Work out the finished part from the listing and answer in its coordinate system (mm). A direction names the side the tool comes from. Give positions to 0.01 mm unless a question says otherwise; leave off trailing zeros. Order: outer loops, then holes, each group sorted by start corner. A loop starts at its lowest first (then second) coordinate and runs counter-clockwise, first axis right, second up.
```python
from build123d import *

# Parameters (mm, degrees)
SKETCH_1_W          = 82
SKETCH_1_H          = 82
SKETCH_1_R          = 35.5
EXTRUDE_1_DEPTH     = 315
SKETCH_2_W          = 82
SKETCH_2_H          = 82
EXTRUDE_2_DEPTH     = 35
SKETCH_3_W          = 8
SKETCH_3_H          = 20
CUT_EXTRUDE_1_DEPTH = 315
SKETCH_4_R          = 4
CUT_EXTRUDE_2_DEPTH = 20
FILLET_2_R          = 3
FILLET_3_R          = 3
FILLET_4_R          = 3
FILLET_5_R          = 3
CUT_EXTRUDE_3_DEPTH = 12
SKETCH_6_W          = 29.4
SKETCH_6_H          = 3
CUT_EXTRUDE_4_DEPTH = 10


with BuildPart() as part:
    # 草圖1 → 填料-伸長1 (new body)
    with BuildSketch(Plane.XY):
        Rectangle(SKETCH_1_W, SKETCH_1_H)
        Circle(SKETCH_1_R, mode=Mode.SUBTRACT)
    extrude(amount=EXTRUDE_1_DEPTH)

    # 草圖2 → 填料-伸長2 (add)
    with BuildSketch(Plane(origin=(0, 0, 0), x_dir=(-1, 0, 0), z_dir=(0, 0, -1))):
        Rectangle(SKETCH_2_W, SKETCH_2_H)
    extrude(amount=EXTRUDE_2_DEPTH)

    # 草圖3 → 除料-伸長1 (cut)
    with BuildSketch(Plane.XY.offset(315)):
        with Locations((-37, 0)):
            Rectangle(SKETCH_3_W, SKETCH_3_H)
    extrude(amount=-CUT_EXTRUDE_1_DEPTH, mode=Mode.SUBTRACT)

    # 草圖4 → 除料-伸長2 (cut)
    with BuildSketch(Plane.XY.offset(315)):
        with Locations((-32.9, 33)):
            Circle(SKETCH_4_R)
        with Locations((33.1, 32.9)):
            Circle(SKETCH_4_R)
        with Locations((33, -33.1)):
            Circle(SKETCH_4_R)
        with Locations((-33, -33)):
            Circle(SKETCH_4_R)
    extrude(amount=-CUT_EXTRUDE_2_DEPTH, mode=Mode.SUBTRACT)

    # 圓角2
    fillet_2_edges = [part.edges().sort_by_distance(p)[0] for p in [
        (-36.9, 33, 295),
    ]]
    fillet(fillet_2_edges, radius=FILLET_2_R)

    # 圓角3
    fillet_3_edges = [part.edges().sort_by_distance(p)[0] for p in [
        (29.1, 32.9, 295),
    ]]
    fillet(fillet_3_edges, radius=FILLET_3_R)

    # 圓角4
    fillet_4_edges = [part.edges().sort_by_distance(p)[0] for p in [
        (-37, -33, 295),
    ]]
    fillet(fillet_4_edges, radius=FILLET_4_R)

    # 圓角5
    fillet_5_edges = [part.edges().sort_by_distance(p)[0] for p in [
        (29, -33.1, 295),
    ]]
    fillet(fillet_5_edges, radius=FILLET_5_R)

    # 草圖5 → 除料-伸長3 (cut)
    with BuildSketch(Plane(origin=(0, 41, 0), x_dir=(1, 0, 0), z_dir=(0, 1, 0))):
        with BuildLine():
            Line((-39, 5), (-39, 30))
            ThreePointArc((-39, 30), (-36.8, 32.2), (-34.6, 30))
            Line((-34.6, 30), (-34.6, 5))
            ThreePointArc((-34.6, 5), (-36.8, 2.8), (-39, 5))
        make_face()
    extrude(amount=-CUT_EXTRUDE_3_DEPTH, mode=Mode.SUBTRACT)

    # 草圖6 → 除料-伸長4 (cut)
    with BuildSketch(Plane.ZY.offset(41)):
        with Locations((-17.5, 34.5)):
            Rectangle(SKETCH_6_W, SKETCH_6_H)
    extrude(amount=-CUT_EXTRUDE_4_DEPTH, mode=Mode.SUBTRACT)


solid = part.part
```
1. Which of the six approach directions +Z, -Z, +X, -X, +Y, -Y give full straight-line access (tool end or side, diameter ignored) to faces 1 (the face through (36, 1, 315)), 2 (the face through (-41, -19, 142)), 3 (the face through (-38, -10, 160)), 4 (the face through (-33, 33, -18)), 5 (the face through (29.8, -35.5, 306.6))?
Findings below:
face 1: +Z, +X, -X, +Y, -Y
face 2: +Z, -Z, -X, +Y, -Y
face 3: +Z, -X
face 4: -X
face 5: +Z
2. The mould has two halves that part along Z. Classify faces 6 (the face through (-3, 0, 0)), 7 (the face through (-33, 36, -18)), 8 (the face through (29.9, 30.5, 306.6)): pulls with the +Z half, pulls with the -Z half, needs draft (parallel to the pull), parting line crosses it, or undercut.
Findings below:
face 6: pulls with the +Z half
face 7: undercut
face 8: needs draft
3. Straight lines are drawn through the part: probe 1 along Y at (x, z) = (33, 302); probe 2 along Z at (x, y) = (10.5, -3); probe 3 along X at (y, z) = (-29, 161.5). For each, find the intervals that lie inside material, in ascending order.
Findings below:
probe 1: y = -41 to -37.1, -29.1 to -13.09, 13.09 to 28.9, 36.9 to 41
probe 2: z = -35 to 0
probe 3: x = -41 to -20.48, 20.48 to 41
4. The part is cut by section C-C (x = 26). Write down the section's boundary in (y, z).
Findings below:
outline: (-41, -35) - (41, -35) - (41, 315) - (24.17, 315) - (24.17, 0) - (-24.17, 0) - (-24.17, 315) - (-41, 315) - close
5. The part is cut by section A-A (y = 0). Write down the section's boundary in (x, z).
Findings below:
outline: (-41, -35) - (41, -35) - (41, 315) - (35.5, 315) - (35.5, 0) - (-41, 0) - close
6. The part is cut by section B-B (z = 27). Write down the section's boundary in (x, y), then the cut area to 3 significant figures.
Findings below:
outline: (-41, -41) - (41, -41) - (41, 41) - (-41, 41) - (-41, 10) - (-34.06, 10) arc R35.5 cw (long way) to (-34.06, -10) - (-41, -10) - close
area: 2,650 mm2
7. Given P1, Ø1.6, axis at x = 33, y = -33, coming from the +Z side; P2, Ø8, axis at y = 0, z = 239, coming from the -X side; P3, Ø2, axis at x = -36, z = -17.5, coming from the +Y side, each flat-ended and moving along its own axis, determine where each tip first touches the part or whether it passes through.
Findings below:
P1: stops at z = 295
P2: stops at x = 35.27
P3: stops at y = 29
